The model under review builds one solid part; all positions refer to its coordinate system, in mm. A direction names the side the tool comes from. Give positions to 0.01 mm unless a question says otherwise; leave off trailing zeros. Loops run counter-clockwise (first coordinate to the right, second up) from the corner with the lowest first, then second, coordinate; pieces in that order, holes last. Notation, with made-up numbers: (33, 74.25) - (81, 74.25) arc R24 cw to (81, 101.25) - close; hole circle Ø8 at (61, -22.5). An arc over 180 degrees is marked (long way). Answer as a JSON object with one key per item and string values.
from build123d import *

# Parameters (mm, degrees)
SKETCH_1_R          = 4
EXTRUDE_1_DEPTH     = 20
SKETCH_2_R          = 1.65
SKETCH_2_R_2        = 1.6
EXTRUDE_2_DEPTH     = 5
SKETCH_3_R          = 2.25
CUT_EXTRUDE_1_DEPTH = 12
SKETCH_4_R          = 2.225
CUT_EXTRUDE_2_DEPTH = 18.59438831
FILLET_2_R          = 1


with BuildPart() as part:
    # 草图1 → 凸台-拉伸1 (new body)
    with BuildSketch(Plane.XY):
        Circle(SKETCH_1_R)
    extrude(amount=EXTRUDE_1_DEPTH)

    # 草图2 → 凸台-拉伸2 (add)
    with BuildSketch(Plane(origin=(0, 0, 0), x_dir=(-1, 0, 0), z_dir=(0, 0, -1))):
        with BuildLine():
            Line((-8.7734375, 2.638994967), (-1.40625, 4.798172666))
            ThreePointArc((-1.40625, 4.798172666), (0, 5), (1.40625, 4.798172666))
            Line((1.40625, 4.798172666), (8.7734375, 2.638994967))
            ThreePointArc((8.7734375, 2.638994967), (10.75, 0), (8.7734375, -2.638994967))
            Line((8.7734375, -2.638994967), (1.40625, -4.798172666))
            ThreePointArc((1.40625, -4.798172666), (0, -5), (-1.40625, -4.798172666))
            Line((-1.40625, -4.798172666), (-8.7734375, -2.638994967))
            ThreePointArc((-8.7734375, -2.638994967), (-10.75, 0), (-8.7734375, 2.638994967))
        make_face()
        with Locations((-8, 0)):
            Circle(SKETCH_2_R, mode=Mode.SUBTRACT)
        with Locations((8, 0)):
            Circle(SKETCH_2_R_2, mode=Mode.SUBTRACT)
    extrude(amount=EXTRUDE_2_DEPTH)

    # 草图3 → 切除-拉伸1 (cut)
    with BuildSketch(Plane(origin=(0, 0, -5), x_dir=(-1, 0, 0), z_dir=(0, 0, -1))):
        Circle(SKETCH_3_R)
    extrude(amount=-CUT_EXTRUDE_1_DEPTH, mode=Mode.SUBTRACT)

    # 草图4 → 切除-拉伸2 (cut, through all)
    with BuildSketch(Plane(origin=(0, 0, 7), x_dir=(-1, 0, 0), z_dir=(0, 0, -1))):
        Circle(SKETCH_4_R)
    extrude(amount=-CUT_EXTRUDE_2_DEPTH, mode=Mode.SUBTRACT)

    # 圆角2
    fillet_2_edges = [part.edges().sort_by_distance(p)[0] for p in [
        (-4, 0, 20),
    ]]
    fillet(fillet_2_edges, radius=FILLET_2_R)


solid = part.part
Q1. Consider section B-B, the plane z = -2.25. State the section outline as (x, y) points, plus the area to 3 significant figures.
Results:
{"outline": "(-8.77, -2.64) - (-1.41, -4.8) arc R5 ccw to (1.41, -4.8) - (8.77, -2.64) arc R2.75 ccw to (8.77, 2.64) - (1.41, 4.8) arc R5 ccw to (-1.41, 4.8) - (-8.77, 2.64) arc R2.75 ccw to start; hole circle Ø3.2 at (-8, 0); hole circle Ø4.5 at (0, 0); hole circle Ø3.3 at (8, 0)", "area": "120 mm^2"}
Q2. Consider section A-A, the plane x = 0. State the section outline as (y, z) points (3 decimals), plus the area to 3 significant figures.
Results:
{"outline": "(-5, -5) - (-2.25, -5) - (-2.25, 7) - (-2.225, 7) - (-2.225, 20) - (-3, 20) arc R1 ccw to (-4, 19) - (-4, 0) - (-5, 0) - close; (2.225, 7) - (2.25, 7) - (2.25, -5) - (5, -5) - (5, 0) - (4, 0) - (4, 19) arc R1 ccw to (3, 20) - (2.225, 20) - close", "area": "97.7 mm^2"}
Q3. For faces 1 (the face through (-0.867, -3.905, 9.367)), 2 (the face through (-6.4, 0.07, -2.46)), list the 3-axis set-ups (+Z, -Z, +X, -X, +Y, -Y) from which the entire face can be reached by the end or side of a thin tool; tool diameter is ignored.
Results:
{"face 1": "+Z", "face 2": "+Z, -Z"}
Q4. To check wall thickness, follow probe 1 along Y at (x, z) = (0, 2.5); probe 2 along X at (y, z) = (-0.5, -0.5); probe 3 along Z at (x, y) = (-3.5, 2.25). State the ranges of each line that lie inside material, in increasing order. Write a range as [from, to].
Results:
{"probe 1": "y = [-4, -2.25], [2.25, 4]", "probe 2": "x = [-10.7, -9.52], [-6.48, -2.19], [2.19, 6.43], [9.57, 10.7]", "probe 3": "z = [-5, 0]"}
Q5. The part is to be moulded in two halves that separate along X. For faces 3 (the face through (5.038, -3.734, -2.465)), 4 (the face through (0.29, 2.23, 0.92)), 5 (the face through (-3, -3, 0)), say which applies: +X half, -X half, draft (parallel to the pull), parting line (faces both ways), or undercut.
Results:
{"face 3": "+X half", "face 4": "undercut", "face 5": "draft"}
Q6. Consider section D-D, the plane x = 9.25. State the section outline as (y, z) points.
Results:
{"outline": "(-2.45, -5) - (-1.08, -5) - (-1.08, 0) - (-2.45, 0) - close; (1.08, -5) - (2.45, -5) - (2.45, 0) - (1.08, 0) - close"}
Q7. Clearance check with flat-ended pins moving along their axes: pin 1 Ø2.5 at (x, y) = (-8, 0) entering from -Z; pin 2 Ø5 at (x, z) = (-0.5, 10) entering from +Y; pin 3 Ø6 at (x, z) = (2, 13.5) entering from -Y; pin 4 Ø1.5 at (x, y) = (-4.5, 0) entering from +Z. State where each tip first meets the part, or that it passes through.
Results:
{"pin 1": "passes through", "pin 2": "stops at y = 4", "pin 3": "stops at y = -4", "pin 4": "stops at z = 19.66"}
Q8. Consider section C-C, the plane y = 0. State the section outline as (x, z) points (3 decimals).
Results:
{"outline": "(-10.75, -5) - (-9.6, -5) - (-9.6, 0) - (-10.75, 0) - close; (-6.4, -5) - (-2.25, -5) - (-2.25, 7) - (-2.225, 7) - (-2.225, 20) - (-3, 20) arc R1 ccw to (-4, 19) - (-4, 0) - (-6.4, 0) - close; (2.225, 7) - (2.25, 7) - (2.25, -5) - (6.35, -5) - (6.35, 0) - (4, 0) - (4, 19) arc R1 ccw to (3, 20) - (2.225, 20) - close; (9.65, -5) - (10.75, -5) - (10.75, 0) - (9.65, 0) - close"}
